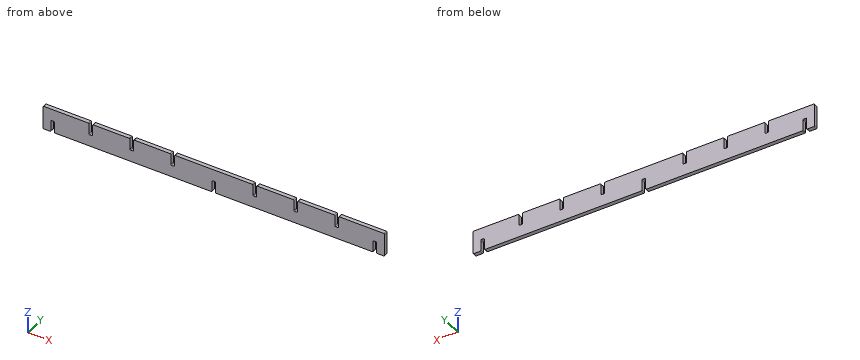
Autodesk Inventor part; units mm, degrees
ref_plane "YZ Plane" through (0, 0, 0) normal (1, 0, 0) x (0, 1, 0)
ref_plane "XZ Plane" through (0, 0, 0) normal (0, 1, 0) x (-1, 0, 0)
ref_plane "XY Plane" through (0, 0, 0) normal (0, 0, 1) x (1, 0, 0)
sketch "Sketch1" plane through (0, 0, 0) normal (0, 1, 0) x (-1, 0, 0)
  line L0 (0, 0) -> (435, 0)
  line L1 (435, 0) -> (435, -30)
  line L2 (435, -30) -> (0, -30)
  line L3 (0, -30) -> (0, 0)
  dimension "d0" = 435
  dimension "d1" = 30
extrude "Extrusion1" add sketch "Sketch1" along normal blind 5
sketch "Sketch2" plane through (0, 5, 0) normal (0, 1, 0) x (1, 0, 0)
  line L0 (0, 30) -> (-435, 30)
  line L1 (-435, 30) -> (-425, 30)
  line L2 (-425, 30) -> (-420.5, 30)
  line L3 (-420.5, 30) -> (-420.5, 15)
  line L4 (-420.5, 15) -> (-425, 15)
  line L5 (-425, 15) -> (-425, 30)
  line L6 (-420.5, 30) -> (-219.75, 30)
  line L7 (-219.75, 30) -> (-215.25, 30)
  line L8 (-215.25, 30) -> (-215.25, 15)
  line L9 (-215.25, 15) -> (-219.75, 15)
  line L10 (-219.75, 15) -> (-219.75, 30)
  line L11 (-215.25, 30) -> (-14.5, 30)
  line L12 (-14.5, 30) -> (-10, 30)
  line L13 (-10, 30) -> (-10, 15)
  line L14 (-10, 15) -> (-14.5, 15)
  line L15 (-14.5, 15) -> (-14.5, 30)
  point P0 (0, 0)
  dimension "d4" = 10
  dimension "d5" = 4.5
  dimension "d6" = 15
  dimension "d7" = 200.75
  dimension "d8" = 4.5
  dimension "d9" = 15
  dimension "d10" = 200.75
  dimension "d11" = 4.5
  dimension "d12" = 15
extrude "Extrusion2" cut sketch "Sketch2" against normal blind 5
sketch "Sketch6" plane through (0, 5, 0) normal (0, 1, 0) x (1, 0, 0)
  line L0 (-14.5, 30) -> (-14.5, 15)
  line L1 (-14.5, 15) -> (-58.5, 15)
  line L2 (-14.5, 30) -> (-215.25, 30)
  line L3 (-58.5, 15) -> (-63, 15)
  line L4 (-63, 15) -> (-63, 30)
  line L5 (-63, 30) -> (-58.5, 30)
  line L6 (-58.5, 30) -> (-58.5, 15)
  line L7 (-63, 15) -> (-110.75, 15)
  line L8 (-110.75, 15) -> (-115.25, 15)
  line L9 (-115.25, 15) -> (-115.25, 30)
  line L10 (-115.25, 30) -> (-110.75, 30)
  line L11 (-110.75, 30) -> (-110.75, 15)
  line L12 (-115.25, 15) -> (-163, 15)
  line L13 (-163, 15) -> (-167.5, 15)
  line L14 (-167.5, 15) -> (-167.5, 30)
  line L15 (-167.5, 30) -> (-163, 30)
  line L16 (-163, 30) -> (-163, 15)
  line L17 (-435, 0) -> (0, 0)
  line L18 (-217.5, 0) -> (-217.5, 47.2454)
  line L19 (-376.5, 15) -> (-372, 15)
  line L20 (-372, 15) -> (-372, 30)
  line L21 (-372, 30) -> (-376.5, 30)
  line L22 (-376.5, 30) -> (-376.5, 15)
  line L23 (-372, 15) -> (-324.25, 15)
  line L24 (-324.25, 15) -> (-319.75, 15)
  line L25 (-319.75, 15) -> (-319.75, 30)
  line L26 (-319.75, 30) -> (-324.25, 30)
  line L27 (-324.25, 30) -> (-324.25, 15)
  line L28 (-319.75, 15) -> (-272, 15)
  line L29 (-272, 15) -> (-267.5, 15)
  line L30 (-267.5, 15) -> (-267.5, 30)
  line L31 (-267.5, 30) -> (-272, 30)
  line L32 (-272, 30) -> (-272, 15)
  line L33 (-110.75, 15) -> (-115.25, 15)
  line L34 (-115.25, 15) -> (-115.25, 0)
  line L35 (-115.25, 0) -> (-110.75, 0)
  line L36 (-110.75, 0) -> (-110.75, 15)
  line L37 (-319.75, 15) -> (-324.25, 15)
  line L38 (-324.25, 15) -> (-324.25, 0)
  line L39 (-324.25, 0) -> (-319.75, 0)
  line L40 (-319.75, 0) -> (-319.75, 15)
  line L41 (-58.5, 0) -> (-63, 0)
  line L42 (-63, 0) -> (-63, 15)
  line L43 (-63, 15) -> (-58.5, 15)
  line L44 (-58.5, 15) -> (-58.5, 0)
  line L45 (-163, 0) -> (-167.5, 0)
  line L46 (-167.5, 0) -> (-167.5, 15)
  line L47 (-167.5, 15) -> (-163, 15)
  line L48 (-163, 15) -> (-163, 0)
  line L49 (-267.5, 15) -> (-272, 15)
  line L50 (-272, 15) -> (-272, 0)
  line L51 (-272, 0) -> (-267.5, 0)
  line L52 (-267.5, 0) -> (-267.5, 15)
  line L53 (-372, 15) -> (-376.5, 15)
  line L54 (-376.5, 15) -> (-376.5, 0)
  line L55 (-376.5, 0) -> (-372, 0)
  line L56 (-372, 0) -> (-372, 15)
  line L57 (-435, 30) -> (-435, 0)
  dimension "d40" = 44
  dimension "d41" = 4.5
  dimension "d42" = 47.75
  dimension "d43" = 4.5
  dimension "d44" = 47.75
  dimension "d45" = 4.5
  dimension "d48" = 15
  dimension "d49" = 4.5
  dimension "d50" = 106.75
  dimension "d51" = 58.5
  dimension "d52" = 54.5
extrude "Extrusion6" cut sketch "Sketch6" against normal blind 5 contours L17 L50 L29 L52 | L44 L17 L42 L3 | L36 L17 L34 L8 | L48 L17 L46 L13 | L17 L38 L24 L40 | L17 L54 L19 L56
fillet "Fillet2" radius 1 40 edges at (-324.25, 2.5, -15) (-319.75, 2.5, -15) (-372, 2.5, -15) (-376.5, 2.5, -15) (-425, 2.5, -15) (-420.5, 2.5, -15) (-267.5, 2.5, -15) (-272, 2.5, -15) (-215.25, 2.5, -15) (-219.75, 2.5, -15) (-167.5, 2.5, -15) (-163, 2.5, -15) (-115.25, 2.5, -15) (-110.75, 2.5, -15) (-63, 2.5, -15) (-58.5, 2.5, -15) (-14.5, 2.5, -15) (-10, 2.5, -15) (-58.5, 2.5, 0) (-63, 2.5, 0) (-110.75, 2.5, 0) (-115.25, 2.5, 0) (-163, 2.5, 0) (-167.5, 2.5, 0) (-215.25, 2.5, -30) (-219.75, 2.5, -30) (-267.5, 2.5, 0) (-272, 2.5, 0) (-319.75, 2.5, 0) (-324.25, 2.5, 0) (-372, 2.5, 0) (-376.5, 2.5, 0) (-435, 2.5, 0) (-435, 2.5, -30) (-425, 2.5, -30) (-420.5, 2.5, -30) (0, 2.5, 0) (-10, 2.5, -30) (-14.5, 2.5, -30) (0, 2.5, -30)
properties part number "slats_under" material "Foam Core Board"
Read the model definition and answer for the solid it produces. Units are mm, in the model's axes. Round coordinates to 2 decimals unless told otherwise and drop trailing zeros. Loops run counter-clockwise (first coordinate to the right, second up) from the corner with the lowest first, then second, coordinate; pieces in that order, holes last.
Q1. Consider probe 1 along X at (y, z) = (1.05, -20.75); probe 2 along X at (y, z) = (4.35, -15.5); probe 3 along Z at (x, y) = (-374, 2.35). Determine where each line is inside the solid, lowest interval first.
Q2. Each of these flat-tipped pins is pushed along its axis until it touches: pin 1 (2 mm diameter, centred on x = -165.5, y = 2.5, fed in from +Z); pin 2 (2 mm diameter, centred on x = -11.5, y = 3, fed in from -Z). Where does it stop, or does it pass through?
Q3. Section A-A on z = -21 is taken. Write down the section's boundary in (x, y), and give its area (3 significant figures).
Output:
1. probe 1: x = -435 to -425, -420.5 to -219.75, -215.25 to -14.5, -10 to 0
1. probe 2: x = -435 to -424.87, -420.63 to -219.62, -215.38 to -14.37, -10.13 to 0
1. probe 3: z = -30 to -15
2. pin 1: stops at z = -15
2. pin 2: stops at z = -15.13
3. outline: (-435, 0) - (-425, 0) - (-425, 5) - (-435, 5) - close; (-420.5, 0) - (-219.75, 0) - (-219.75, 5) - (-420.5, 5) - close; (-215.25, 0) - (-14.5, 0) - (-14.5, 5) - (-215.25, 5) - close; (-10, 0) - (0, 0) - (0, 5) - (-10, 5) - close
3. area: 2,110 mm2
